Work out the finished part from the listing and answer in its coordinate system (mm). Face numbers are marked on the shaded views. A direction names the side the tool comes from. Give positions to 0.01 mm unless a question says otherwise; leave off trailing zeros. Order: outer loops, then holes, each group sorted by start corner. A loop starts at its lowest first (then second) coordinate and runs counter-clockwise, first axis right, second up. Notation, with made-up numbers: (52.5, 8.25) - (68.5, 8.25) arc R24 cw to (68.5, 38.25) - close; hole circle Ø1 at (67.25, 27.5). An arc over 180 degrees is marked (long way). Put each result on its own line as item: value.
```python
from build123d import *

# Parameters (mm, degrees)
SKETCH1_W           = 42
SKETCH1_H           = 28
SKETCH1_R           = 6
BOSS_EXTRUDE1_DEPTH = 18
CUT_EXTRUDE5_DEPTH  = 37
SKETCH2_R           = 2.15
CUT_EXTRUDE1_DEPTH  = 29
SKETCH3_R           = 2.5
CUT_EXTRUDE2_DEPTH  = 12
SKETCH4_R           = 11
CUT_EXTRUDE3_DEPTH  = 1
SKETCH5_R           = 11
CUT_EXTRUDE4_DEPTH  = 1


with BuildPart() as part:
    # Sketch1 → Boss-Extrude1 (new body, symmetric)
    with BuildSketch(Plane.XY):
        Rectangle(SKETCH1_W, SKETCH1_H)
        with Locations((0, -1)):
            Circle(SKETCH1_R, mode=Mode.SUBTRACT)
    extrude(amount=BOSS_EXTRUDE1_DEPTH, both=True)

    # Sketch6 → Cut-Extrude5 (cut, through all)
    with BuildSketch(Plane.XY.offset(18)):
        Polygon((-21, -9), (-9, -9), (-4.804501844, -14), (-21, -14), align=None)
        Polygon((21, -9), (9, -9), (4, -14), (21, -14), align=None)
    extrude(amount=-CUT_EXTRUDE5_DEPTH, mode=Mode.SUBTRACT)

    # Sketch2 → Cut-Extrude1 (cut, through all)
    with BuildSketch(Plane(origin=(0, 14, 0), x_dir=(-1, 0, 0), z_dir=(0, -1, 0))):
        with Locations((15.25, -13)):
            Circle(SKETCH2_R)
        with Locations((-15.25, -13)):
            Circle(SKETCH2_R)
        with Locations((-15.25, 13)):
            Circle(SKETCH2_R)
        with Locations((15.25, 13)):
            Circle(SKETCH2_R)
    extrude(amount=CUT_EXTRUDE1_DEPTH, mode=Mode.SUBTRACT)

    # Sketch3 → Cut-Extrude2 (cut)
    with BuildSketch(Plane.XZ.offset(-14)):
        with Locations((-15.25, 13)):
            Circle(SKETCH3_R)
        with Locations((15.25, 13)):
            Circle(SKETCH3_R)
        with Locations((15.25, -13)):
            Circle(SKETCH3_R)
        with Locations((-15.25, -13)):
            Circle(SKETCH3_R)
    extrude(amount=CUT_EXTRUDE2_DEPTH, mode=Mode.SUBTRACT)

    # Sketch4 → Cut-Extrude3 (cut)
    with BuildSketch(Plane.XY.offset(18)):
        with Locations((0, -1)):
            Circle(SKETCH4_R)
    extrude(amount=-CUT_EXTRUDE3_DEPTH, mode=Mode.SUBTRACT)

    # Sketch5 → Cut-Extrude4 (cut)
    with BuildSketch(Plane(origin=(0, 0, -18), x_dir=(-1, 0, 0), z_dir=(0, 0, -1))):
        with Locations((0, -1)):
            Circle(SKETCH5_R)
    extrude(amount=-CUT_EXTRUDE4_DEPTH, mode=Mode.SUBTRACT)


solid = part.part
```
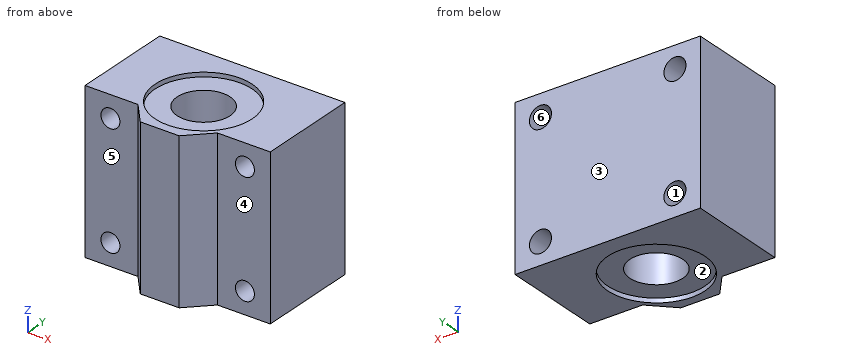
(1) Straight lines are drawn through the part: line 1 (Z direction, x = 15, y = 3.5); line 2 (Y direction, x = 0, z = 17.75); line 3 (X direction, y = -2.75, z = 12). For each, find the intervals that lie inside material, in ascending order.
Geometry check:
line 1: z = -18 to -15.49, -10.51 to 10.51, 15.49 to 18
line 2: y = -14 to -12, 10 to 14
line 3: x = -21 to -17.15, -13.35 to -5.74, 5.74 to 13.35, 17.15 to 21
(2) Section D-D, the plane x = 0 is taken. Write down the section's boundary in (y, z).
Geometry check:
outline: (-14, -18) - (-12, -18) - (-12, -17) - (-7, -17) - (-7, 17) - (-12, 17) - (-12, 18) - (-14, 18) - close; (5, -17) - (10, -17) - (10, -18) - (14, -18) - (14, 18) - (10, 18) - (10, 17) - (5, 17) - close
(3) Given pin 1 (5 mm diameter, centred on x = 15.25, z = 13, fed in from -Y); pin 2 (15.5 mm diameter, centred on x = 0, y = -1, fed in from +Z), each flat-ended and moving along its own axis, determine where each tip first touches the part or whether it passes through.
Geometry check:
pin 1: stops at y = -9
pin 2: stops at z = 17
(4) A tool of negligible diameter and unlimited length cuts with its end or side. For the marked faces 4, 5 and 6, from which of +Z, -Z, +X, -X, +Y, -Y can it reach the whole face along a straight path? Write none if from no direction.
Geometry check:
face 4: +Z, -Z, +X, -Y
face 5: +Z, -Z, -X, -Y
face 6: +Y
(5) Determine the mould class of the marked faces 1, 2 and 3 for opening direction Y: pulls with the +Y half, pulls with the -Y half, needs draft (parallel to the pull), parting line crosses it, or undercut.
Geometry check:
face 1: needs draft
face 2: undercut
face 3: pulls with the +Y half
(6) Section B-B, the plane x = -15.25 is taken. Write down the section's boundary in (y, z), then the cut area to 3 significant figures.
Geometry check:
outline: (-9, -18) - (14, -18) - (14, -15.5) - (2, -15.5) - (2, -15.15) - (-9, -15.15) - close; (-9, -10.85) - (2, -10.85) - (2, -10.5) - (14, -10.5) - (14, 10.5) - (2, 10.5) - (2, 10.85) - (-9, 10.85) - close; (-9, 15.15) - (2, 15.15) - (2, 15.5) - (14, 15.5) - (14, 18) - (-9, 18) - close
area: 613 mm²
(7) Section A-A, the plane z = 13 is taken. Write down the section's boundary in (x, y), then the cut area to 3 significant figures.
Geometry check:
outline: (-21, -9) - (-17.4, -9) - (-17.4, 2) - (-17.75, 2) - (-17.75, 14) - (-21, 14) - close; (-13.1, -9) - (-9, -9) - (-4.8, -14) - (4, -14) - (9, -9) - (13.1, -9) - (13.1, 2) - (12.75, 2) - (12.75, 14) - (-12.75, 14) - (-12.75, 2) - (-13.1, 2) - close; (17.4, -9) - (21, -9) - (21, 14) - (17.75, 14) - (17.75, 2) - (17.4, 2) - close; hole circle Ø12 at (0, -1)
area: 705 mm²
(8) Section C-C, the plane y = -3.75 is taken. Write down the section's boundary in (x, z).
Geometry check:
outline: (-21, -18) - (-10.65, -18) - (-10.65, -17) - (-5.33, -17) - (-5.33, 17) - (-10.65, 17) - (-10.65, 18) - (-21, 18) - close; (5.33, -17) - (10.65, -17) - (10.65, -18) - (21, -18) - (21, 18) - (10.65, 18) - (10.65, 17) - (5.33, 17) - close; hole circle Ø4.3 at (-15.25, -13); hole circle Ø4.3 at (-15.25, 13); hole circle Ø4.3 at (15.25, -13); hole circle Ø4.3 at (15.25, 13)
